Autodesk Inventor part; units mm, degrees
ref_plane "YZ Plane" through (0, 0, 0) normal (1, 0, 0) x (0, 1, 0)
ref_plane "XZ Plane" through (0, 0, 0) normal (0, 1, 0) x (-1, 0, 0)
ref_plane "XY Plane" through (0, 0, 0) normal (0, 0, 1) x (1, 0, 0)
sketch "Boceto1" plane through (0, 0, 0) normal (0, 0, 1) x (1, 0, 0)
  line L0 (-116.5, 26.5) -> (-116.5, -26.5)
  line L1 (-1.5, 26.5) -> (-1.5, -26.5)
  line L2 (-116.5, -26.5) -> (-1.5, -26.5)
  line L3 (-1.5, -26.5) -> (-1.5, 26.5)
  line L4 (-1.5, 26.5) -> (-116.5, 26.5)
  line L5 (-116.5, 26.5) -> (-116.5, -26.5)
  point P0 (0, 0)
extrude "interior" add sketch "Boceto1" against normal blind 3
sketch "Boceto2" plane through (0, 0, 0) normal (0, 0, 1) x (1, 0, 0)
  line L0 (-119.5, -31.5) -> (-119.5, 31.5)
  line L1 (1.5, -31.5) -> (1.5, 31.5)
  line L2 (-119.5, -31.5) -> (1.5, -31.5)
  line L3 (1.5, -31.5) -> (1.5, 31.5)
  line L4 (1.5, 31.5) -> (-119.5, 31.5)
  line L5 (-119.5, 31.5) -> (-119.5, -31.5)
  point P0 (0, 0)
extrude "superior" add sketch "Boceto2" along normal blind 3
sketch "Boceto3" plane through (0, 0, 3) normal (0, 0, 1) x (1, 0, 0)
  line L0 (-119.5, -31.5) -> (1.5, -31.5)
  line L1 (1.5, -31.5) -> (1.5, 31.5)
  line L2 (1.5, 31.5) -> (-119.5, 31.5)
  line L3 (-119.5, 31.5) -> (-119.5, -31.5)
  line L4 (-122.5, 34.5) -> (4.5, 34.5)
  line L5 (4.5, 34.5) -> (4.5, -34.5)
  line L6 (4.5, -34.5) -> (-122.5, -34.5)
  line L7 (-122.5, -34.5) -> (-122.5, 34.5)
  point P0 (0, 0)
  dimension "d4" = 3
extrude "laterales" add sketch "Boceto3" against normal blind 18
sketch "Boceto4" plane through (4.5, -34.5, 3) normal (1, 0, 0) x (0, 0, -1)
  circle A0 centre (11.0023, 11) radius 3
  circle A1 centre (11.0023, 58) radius 2.5
  point P0 (3, 34.5)
hole "Agujero1" at (4.5, -23.5, -8.0023) at (4.5, 23.5, -8.0023) direction (-1, 0, 0) diameter 5 depth 3
ref_plane "Plano de trabajo1" through (-59, -34.5, 3) normal (1, 0, 0) x (0, 0, -1)
mirror "Simetría1" about plane through (-59, -34.5, 3) normal (1, 0, 0) of "Agujero1"
sketch "Boceto5" plane through (0, 0, 3) normal (0, 0, 1) x (1, 0, 0)
  circle A0 centre (1.5, -32) radius 1.25
  circle A1 centre (1.5, -11.7293) radius 1.25
  point P0 (0, 0)
hole "Agujero2" at (1.5, -11.7293, 3) at (1.5, -32, 3) direction (0, 0, -1) diameter 2.5 depth 5 tip angle 118
sketch "Boceto6" plane through (0, 0, 3) normal (0, 0, 1) x (1, 0, 0)
  circle A0 centre (-108.0086, -4.2586) radius 1
  circle A1 centre (-93.4586, -18.4086) radius 1
  point P0 (0, 0)
hole "Agujero3" at (-108.0086, -4.2586, 3) at (-93.4586, -18.4086, 3) direction (0, 0, -1) diameter 2 depth 5 tip angle 118
fillet "Empalme1" radius 2 7 edges at (-116.5, -26.5, -1.5) (-116.5, 26.5, -1.5) (-1.5, 26.5, -1.5) (-1.5, -26.5, -1.5) (1.5, 31.5, -7.5) (-119.5, -31.5, -7.5) (-119.5, 31.5, -7.5)
properties part number "tapa"
For this review, take the finished solid that the model builds, in its own axes (mm). A direction names the side the tool comes from. Coordinates: 2 decimals unless noted, no trailing zeros. Loops run counter-clockwise (first coordinate to the right, second up) from the corner with the lowest first, then second, coordinate; pieces in that order, holes last. Notation, with made-up numbers: (25, 74.25) - (62, 74.25) arc R12 ccw to (62, 91.25) - close; hole circle Ø9 at (87, 71.25). An arc over 180 degrees is marked (long way). Use a Markdown table: item, result. Add a question column.
Item 1: We need section B-B (x = -72.5). Give the boundary of the cut face in (y, z).
Item 2: We need section C-C (y = -8). Give the boundary of the cut face in (x, z).
Item 3: For line 1 (Y direction, x = -46, z = -2.5); line 2 (X direction, y = -15.5, z = -8); line 3 (Y direction, x = -89, z = -5.25), list the stretches that pass through material, from the lowest coordinate up.
Item 4: Tool access review of faces 4 (the face through (-116.5, 0, -1)), 5 (the face through (-64, -33, -15)), 6 (the face through (2.72, -11.46, 1.02)): name each direction out of +Z, -Z, +X, -X, +Y, -Y from which nothing blocks a thin tool from reaching the whole face with its end or side.
Item 5: Insertion check: pin 1 Ø1 at (x, y) = (-99.5, 7) entering from -Z; pin 2 Ø4 at (y, z) = (23.5, -8) entering from -X. Each pin has a flat end and moves straight along its axis. Give the tip position at first contact, or say it passes through.
Item 6: Mouldability with a two-part tool opening along Z and no side actions: class faces 1 (the face through (-64, -28, 0)), 2 (the face through (3, 21, -8)), 3 (the face through (-60, 34.5, -6)) as pulls with the +Z half, pulls with the -Z half, needs draft (parallel to the pull), parting line crosses it, or undercut.
Item 7: We need section A-A (z = -12.5). Give the boundary of the cut face in (x, y).
Results list:
| question | item | result |
|---|---|---|
| 1 | outline | (-34.5, -15) - (-31.5, -15) - (-31.5, 0) - (-26.5, 0) - (-26.5, -3) - (26.5, -3) - (26.5, 0) - (31.5, 0) - (31.5, -15) - (34.5, -15) - (34.5, 3) - (-34.5, 3) - close |
| 2 | outline | (-122.5, -15) - (-119.5, -15) - (-119.5, 0) - (-116.5, 0) - (-116.5, -3) - (-1.5, -3) - (-1.5, 0) - (1.5, 0) - (1.5, -15) - (4.5, -15) - (4.5, 3) - (-122.5, 3) - close |
| 3 | line 1 | y = -34.5 to -31.5, -26.5 to 26.5, 31.5 to 34.5 |
| 3 | line 2 | x = -122.5 to -119.5, 1.5 to 4.5 |
| 3 | line 3 | y = -34.5 to -31.5, 31.5 to 34.5 |
| 4 | face 4 | -Z |
| 4 | face 5 | -Z, +X, -X, +Y, -Y |
| 4 | face 6 | +Z |
| 5 | pin 1 | stops at z = -3 |
| 5 | pin 2 | passes through |
| 6 | face 1 | pulls with the -Z half |
| 6 | face 2 | undercut |
| 6 | face 3 | needs draft |
| 7 | outline | (-122.5, -34.5) - (4.5, -34.5) - (4.5, 34.5) - (-122.5, 34.5) - close; hole (-119.5, -29.5) arc R2 ccw to (-117.5, -31.5) - (1.5, -31.5) - (1.5, 29.5) arc R2 ccw to (-0.5, 31.5) - (-117.5, 31.5) arc R2 ccw to (-119.5, 29.5) - close |
